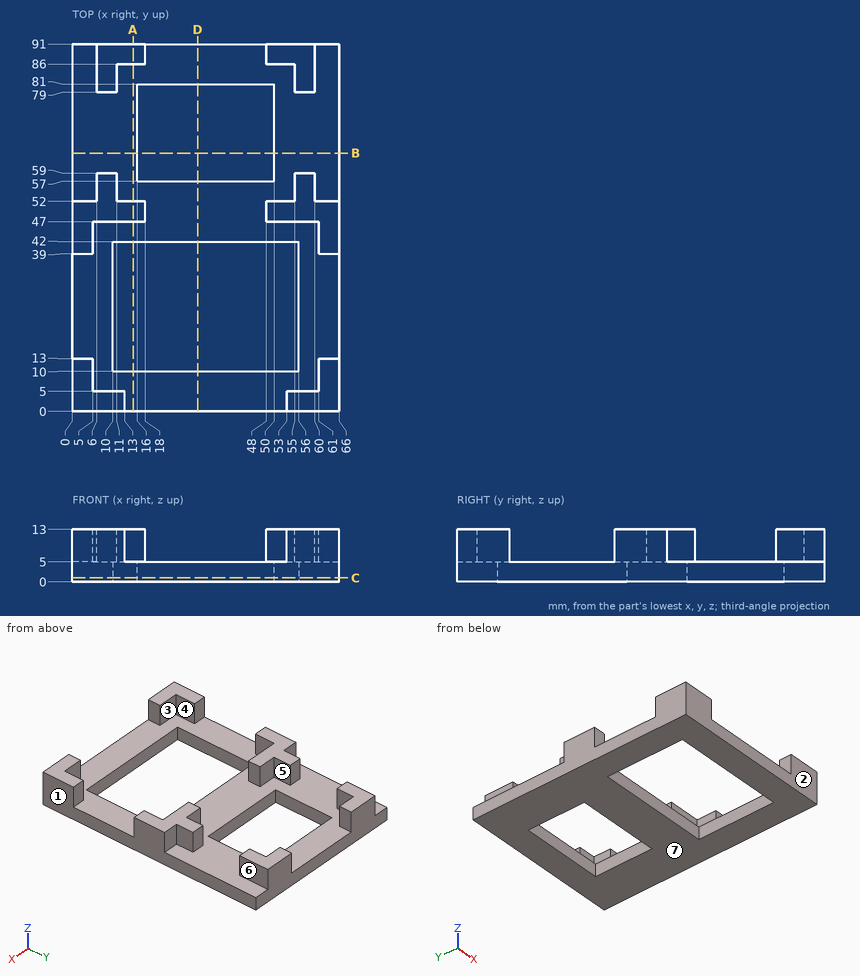
The drawing under review shows one solid part. Ordinate dimensions are in mm from its lowest x, y, z. A direction names the side the tool comes from. Coordinates: 2 decimals unless noted, no trailing zeros. Write each loop counter-clockwise with the first axis right and the second up, starting at its lowest first coordinate (ties: lowest second). Pieces come first, ordered by that corner, then holes. Notation, with made-up numbers: (84.5, 52) - (131.5, 52) arc R20 ccw to (131.5, 84) - close; hole circle Ø1 at (-1.75, 29.25). An arc over 180 degrees is marked (long way). Answer as CSV lines item,"result".
(1) We need section D-D (x = 31). Give the boundary of the cut face in (y, z), plus the area to 3 significant figures.
Data:
outline,"(0, 0) - (10, 0) - (10, 5) - (0, 5) - close; (42, 0) - (57, 0) - (57, 5) - (42, 5) - close; (81, 0) - (91, 0) - (91, 5) - (81, 5) - close"
area,"175 mm2"
(2) Clearance check with flat-ended pins moving along their axes: pin 1 Ø1.5 at (y, z) = (89.5, 8) entering from -X; pin 2 Ø4 at (x, z) = (3.5, 7.5) entering from -Y; pin 3 Ø3 at (x, z) = (4, 11) entering from +Y; pin 4 Ø5.5 at (y, z) = (87.5, 10.5) entering from +X. State where each tip first meets the part, or that it passes through.
Data:
pin 1,"stops at x = 6"
pin 2,"stops at y = 0"
pin 3,"stops at y = 52"
pin 4,"stops at x = 60"
(3) We need section C-C (z = 1). Give the boundary of the cut face in (x, y).
Data:
outline,"(0, 0) - (66, 0) - (66, 91) - (0, 91) - close; hole (10, 10) - (56, 10) - (56, 42) - (10, 42) - close; hole (16, 57) - (50, 57) - (50, 81) - (16, 81) - close"
(4) Tool access review of the marked faces 5, 6 and 7: name each direction out of +Z, -Z, +X, -X, +Y, -Y from which nothing blocks a thin tool from reaching the whole face with its end or side.
Data:
face 5,"+Z"
face 6,"+Z, +X, +Y"
face 7,"-Z, +X, -X, +Y, -Y"
(5) For line 1 along Y through (x, z) = (17, 0.5); line 2 along X through (y, z) = (85, 9.25); line 3 along X through (y, z) = (75.5, 3.25), list the stretches that pass through material, from the lowest coordinate up. Write a range as [from, to].
Data:
line 1,"y = [0, 10], [42, 57], [81, 91]"
line 2,"x = [6, 11], [55, 60]"
line 3,"x = [0, 16], [50, 66]"
(6) We need section A-A (x = 15). Give the boundary of the cut face in (y, z), plus the area to 3 significant figures.
Data:
outline,"(0, 0) - (10, 0) - (10, 5) - (0, 5) - close; (42, 0) - (91, 0) - (91, 13) - (86, 13) - (86, 5) - (52, 5) - (52, 13) - (47, 13) - (47, 5) - (42, 5) - close"
area,"375 mm2"
(7) We need section B-B (y = 64). Give the boundary of the cut face in (x, z).
Data:
outline,"(0, 0) - (16, 0) - (16, 5) - (0, 5) - close; (50, 0) - (66, 0) - (66, 5) - (50, 5) - close"
(8) Mouldability with a two-part tool opening along Y and no side actions: class the marked faces 1, 2, 3 and 4 as pulls with the +Y half, pulls with the -Y half, needs draft (parallel to the pull), parting line crosses it, or undercut.
Data:
face 1,"needs draft"
face 2,"pulls with the -Y half"
face 3,"undercut"
face 4,"undercut"
